Design review of the part built by this model. Coordinates are the model's own, in mm. Round coordinates to 2 decimals unless told otherwise and drop trailing zeros. Loops run counter-clockwise (first coordinate to the right, second up) from the corner with the lowest first, then second, coordinate; pieces in that order, holes last. Notation, with made-up numbers: M 22.25,-16.5 L 31.25,-16.5 A14 ccw 31.25,4.5 Z; hole C 10,-37.5 d5. An arc over 180 degrees is marked long. Use a Markdown table: item, result.
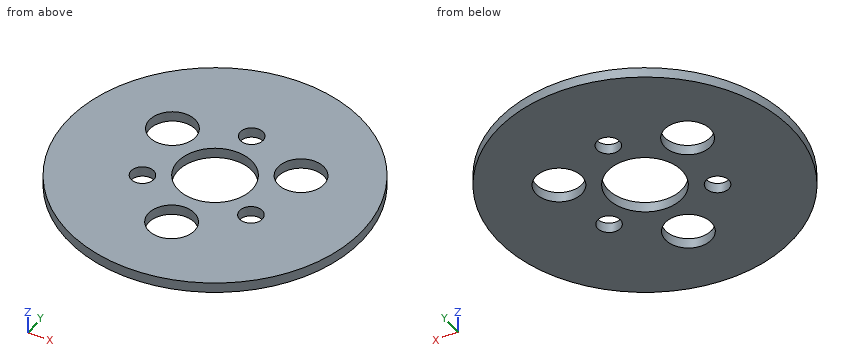
from build123d import *

# Parameters (mm, degrees)
SKETCH1_R           = 57.5
SKETCH1_R_2         = 14.5
SKETCH1_R_3         = 4.445
SKETCH1_R_4         = 9
BOSS_EXTRUDE1_DEPTH = 2


with BuildPart() as part:
    # Sketch1 → Boss-Extrude1 (new body, symmetric)
    with BuildSketch(Plane.XY):
        Circle(SKETCH1_R)
        Circle(SKETCH1_R_2, mode=Mode.SUBTRACT)
        with Locations((0, 24.248711306)):
            Circle(SKETCH1_R_3, mode=Mode.SUBTRACT)
        with Locations((-21, -12.124355653)):
            Circle(SKETCH1_R_3, mode=Mode.SUBTRACT)
        with Locations((21, -12.124355653)):
            Circle(SKETCH1_R_3, mode=Mode.SUBTRACT)
        with Locations((-24.898230359, 14.375)):
            Circle(SKETCH1_R_4, mode=Mode.SUBTRACT)
        with Locations((24.898230359, 14.375)):
            Circle(SKETCH1_R_4, mode=Mode.SUBTRACT)
        with Locations((0, -28.75)):
            Circle(SKETCH1_R_4, mode=Mode.SUBTRACT)
    extrude(amount=BOSS_EXTRUDE1_DEPTH, both=True)


solid = part.part
1. Take a section at A-A on y = 0. Give the boundary of the cut face in (x, z), and give its area (3 significant figures).
Check values:
| item | result |
|---|---|
| outline | M -57.5,-2 L -14.5,-2 L -14.5,2 L -57.5,2 Z; M 14.5,-2 L 57.5,-2 L 57.5,2 L 14.5,2 Z |
| area | 344 mm² |
2. Wall thickness on line 1 along Y through (x, z) = (0, 0.7); line 2 along Y through (x, z) = (-24, -0.9); line 3 along Y through (x, z) = (1, -1.55): over which ranges is each line inside the solid? List them lowest first. Write a range as from..to.
Check values:
| item | result |
|---|---|
| line 1 | y = -57.5..-37.75, -19.75..-14.5, 14.5..19.8, 28.69..57.5 |
| line 2 | y = -52.25..-15.4, -8.84..5.42, 23.33..52.25 |
| line 3 | y = -57.49..-37.69, -19.81..-14.47, 14.47..19.92, 28.58..57.49 |
3. Take a section at C-C on z = -0.6. Give the boundary of the cut face in (x, y) (3 decimals).
Check values:
| item | result |
|---|---|
| outline | C 0,0 d115; hole C -24.898,14.375 d18; hole C -21,-12.124 d8.89; hole C 0,0 d29; hole C 0,-28.75 d18; hole C 0,24.249 d8.89; hole C 24.898,14.375 d18; hole C 21,-12.124 d8.89 |
4. Insertion check: pin 1 (1.5 mm diameter, centred on x = -33, z = -1, fed in from -Y); pin 2 (2 mm diameter, centred on x = -31, z = 0, fed in from +Y). Each pin has a flat end and moves straight along its axis. Give the tip position at first contact, or say it passes through.
Check values:
| item | result |
|---|---|
| pin 1 | stops at y = -47.6 |
| pin 2 | stops at y = 49.05 |
5. Take a section at D-D on x = -29. Give the boundary of the cut face in (y, z), and give its area (3 significant figures).
Check values:
| item | result |
|---|---|
| outline | M -49.65,-2 L 6.36,-2 L 6.36,2 L -49.65,2 Z; M 22.39,-2 L 49.65,-2 L 49.65,2 L 22.39,2 Z |
| area | 333 mm² |
6. Take a section at B-B on x = 0. Give the boundary of the cut face in (y, z), and give its area (3 significant figures).
Check values:
| item | result |
|---|---|
| outline | M -57.5,-2 L -37.75,-2 L -37.75,2 L -57.5,2 Z; M -19.75,-2 L -14.5,-2 L -14.5,2 L -19.75,2 Z; M 14.5,-2 L 19.8,-2 L 19.8,2 L 14.5,2 Z; M 28.69,-2 L 57.5,-2 L 57.5,2 L 28.69,2 Z |
| area | 236 mm² |
